CAD build for the part. Positions are in the model's coordinates, mm. A direction names the side the tool comes from. Coordinates: 2 decimals unless noted, no trailing zeros. Loops run counter-clockwise (first coordinate to the right, second up) from the corner with the lowest first, then second, coordinate; pieces in that order, holes last. Notation, with made-up numbers: (50.5, 62) -> (72.5, 62) arc R27 ccw to (72.5, 90) -> close; hole circle Ø9 at (67, -32.5). An arc over 180 degrees is marked (long way). Write each question's results on one line, items separated by ' | '.
from build123d import *

# Parameters (mm, degrees)
SKETCH1_W           = 66.04
SKETCH1_H           = 38.1
BOSS_EXTRUDE3_DEPTH = 17.78
SKETCH3_W           = 60.96
SKETCH3_H           = 33.02
CUT_EXTRUDE1_DEPTH  = 15.24
SKETCH4_W           = 38.1
SKETCH4_H           = 8.89
CUT_EXTRUDE2_DEPTH  = 66.04
SKETCH5_R           = 0.635
CUT_EXTRUDE3_DEPTH  = 5.08
CUT_EXTRUDE5_DEPTH  = 2.54
FILLET1_R           = 2.54
SKETCH7_R           = 1.5875
CUT_EXTRUDE6_DEPTH  = 1.27


with BuildPart() as part:
    # Sketch1 → Boss-Extrude3 (new body)
    with BuildSketch(Plane(origin=(0, 0, 0), x_dir=(1, 0, 0), z_dir=(0, 1, 0))):
        with Locations((33.02, 19.05)):
            Rectangle(SKETCH1_W, SKETCH1_H)
    extrude(amount=BOSS_EXTRUDE3_DEPTH)

    # Sketch3 → Cut-Extrude1 (cut)
    with BuildSketch(Plane(origin=(0, 17.78, 0), x_dir=(1, 0, 0), z_dir=(0, 1, 0))):
        with Locations((33.02, 19.05)):
            Rectangle(SKETCH3_W, SKETCH3_H)
    extrude(amount=-CUT_EXTRUDE1_DEPTH, mode=Mode.SUBTRACT)

    # Sketch4 → Cut-Extrude2 (cut)
    with BuildSketch(Plane(origin=(66.04, 0, 0), x_dir=(0, 0, -1), z_dir=(1, 0, 0))):
        with Locations((19.05, 13.335)):
            Rectangle(SKETCH4_W, SKETCH4_H)
    extrude(amount=-CUT_EXTRUDE2_DEPTH, mode=Mode.SUBTRACT)

    # Sketch5 → Cut-Extrude3 (cut)
    with BuildSketch(Plane(origin=(0, 8.89, 0), x_dir=(1, 0, 0), z_dir=(0, 1, 0))):
        with Locations((33.02, 36.83)):
            Circle(SKETCH5_R)
        with Locations((33.02, 1.27)):
            Circle(SKETCH5_R)
        with Locations((1.27, 19.05)):
            Circle(SKETCH5_R)
        with Locations((64.77, 19.05)):
            Circle(SKETCH5_R)
    extrude(amount=-CUT_EXTRUDE3_DEPTH, mode=Mode.SUBTRACT)

    # Sketch6 → Cut-Extrude5 (cut)
    with BuildSketch(Plane.ZY):
        with BuildLine():
            Line((-22.86, 7.62), (-15.24, 7.62))
            ThreePointArc((-15.24, 7.62), (-13.335, 5.715), (-15.24, 3.81))
            Line((-15.24, 3.81), (-22.86, 3.81))
            ThreePointArc((-22.86, 3.81), (-24.765, 5.715), (-22.86, 7.62))
        make_face()
    extrude(amount=-CUT_EXTRUDE5_DEPTH, mode=Mode.SUBTRACT)

    # Fillet1
    fillet1_edges = [part.edges().sort_by_distance(p)[0] for p in [
        (33.02, 0, -38.1),
        (66.04, 0, -19.05),
        (33.02, 0, 0),
        (0, 0, -19.05),
    ]]
    fillet(fillet1_edges, radius=FILLET1_R)

    # Sketch7 → Cut-Extrude6 (cut)
    with BuildSketch(Plane.XZ):
        with Locations((33.02, -30.48)):
            Circle(SKETCH7_R)
    extrude(amount=-CUT_EXTRUDE6_DEPTH, mode=Mode.SUBTRACT)


solid = part.part
1) Slice it at C-C (y = 8.25). Write the cut outline in (x, z) (3 decimals), then the cut area to 3 significant figures.
Outcome:
outline: (0, -38.1) -> (66.04, -38.1) -> (66.04, 0) -> (0, 0) -> close; hole circle Ø1.27 at (1.27, -19.05); hole (2.54, -35.56) -> (63.5, -35.56) -> (63.5, -2.54) -> (2.54, -2.54) -> close; hole circle Ø1.27 at (33.02, -36.83); hole circle Ø1.27 at (33.02, -1.27); hole circle Ø1.27 at (64.77, -19.05) | area: 498 mm^2
2) Slice it at A-A (z = -19.05). Write the cut outline in (x, y) (3 decimals), then the cut area to 3 significant figures.
Outcome:
outline: (0, 2.54) arc R2.54 ccw to (2.54, 0) -> (63.5, 0) arc R2.54 ccw to (66.04, 2.54) -> (66.04, 8.89) -> (65.405, 8.89) -> (65.405, 3.81) -> (64.135, 3.81) -> (64.135, 8.89) -> (63.5, 8.89) -> (63.5, 2.54) -> (2.54, 2.54) -> (2.54, 3.81) -> (0, 3.81) -> close; (0, 7.62) -> (0.635, 7.62) -> (0.635, 8.89) -> (0, 8.89) -> close; (1.905, 7.62) -> (2.54, 7.62) -> (2.54, 8.89) -> (1.905, 8.89) -> close | area: 179 mm^2
3) Two-plate mould, pull along Z, no slides. Class faces 4 (the flat face through (33, 6, 0)), 5 (the cylindrical face through (32.386, 6.386, -1.298)), 6 (the flat face through (38, 8.89, -2)): pulls with the +Z half, pulls with the -Z half, needs draft (parallel to the pull), parting line crosses it, or undercut.
Outcome:
face 4: pulls with the +Z half | face 5: undercut | face 6: needs draft
4) Pin check, flat tips, straight feed: pin 1 (3 mm diameter, centred on x = 48, y = 5, fed in from +Z); pin 2 (1 mm diameter, centred on x = 33.02, z = -36.83, fed in from -Y); pin 3 (6 mm diameter, centred on x = 39.5, z = -21, fed in from +Y); pin 4 (1.1 mm diameter, centred on x = 33.02, z = -1.27, fed in from +Y). Stop position of each tip, or through.
Outcome:
pin 1: stops at z = 0 | pin 2: stops at y = 0.12 | pin 3: stops at y = 2.54 | pin 4: stops at y = 3.81
5) Slice it at B-B (x = 33.02). Write the cut outline in (y, z) (1 decimal), then the cut area to 3 significant figures.
Outcome:
outline: (0, -35.6) arc R2.5 ccw to (2.5, -38.1) -> (8.9, -38.1) -> (8.9, -37.5) -> (3.8, -37.5) -> (3.8, -36.2) -> (8.9, -36.2) -> (8.9, -35.6) -> (2.5, -35.6) -> (2.5, -2.5) -> (8.9, -2.5) -> (8.9, -1.9) -> (3.8, -1.9) -> (3.8, -0.6) -> (8.9, -0.6) -> (8.9, 0) -> (2.5, 0) arc R2.5 ccw to (0, -2.5) -> (0, -28.9) -> (1.3, -28.9) -> (1.3, -32.1) -> (0, -32.1) -> close | area: 109 mm^2
6) Slice it at D-D (z = -6). Write the cut outline in (x, y).
Outcome:
outline: (0, 2.54) arc R2.54 ccw to (2.54, 0) -> (63.5, 0) arc R2.54 ccw to (66.04, 2.54) -> (66.04, 8.89) -> (63.5, 8.89) -> (63.5, 2.54) -> (2.54, 2.54) -> (2.54, 8.89) -> (0, 8.89) -> close
7) Drill centre lines: L1, parallel to X at y = 7.85, z = -19.05 (3 decimals); L2, parallel to Z at x = 33.02, y = 6.1 (3 decimals); L3, parallel to Z at x = 17, y = 5.25. Where is each one in solid material? Low to high. Write a range as from..to.
Outcome:
L1: x = 0..0.635, 1.905..2.54, 63.5..64.135, 65.405..66.04 | L2: z = -38.1..-37.465, -36.195..-35.56, -2.54..-1.905, -0.635..0 | L3: z = -38.1..-35.56, -2.54..0
8) Which spindle directions (+Z, -Z, +X, -X, +Y, -Y) get a long thin tool onto all of the face, cutting with end or side? Do faces 1 (the cylindrical face through (1.252, 5.673, -24.765)), 2 (the cylindrical face through (65.276, 0.724, -19.317)), 3 (the cylindrical face through (1.13, 8.26, -18.43)). Say none if no direction does.
Outcome:
face 1: -X | face 2: +Z, -Z, +X, -Y | face 3: +Y
